from build123d import *

# Parameters (mm, degrees)
F0_W        = 127
F0_H        = 622.3
F1_DEPTH    = 19.05
F3_DEPTH    = 622.301
F5_D        = 12.7
F6_W        = 28.575
F6_H        = 28.575
F7_DEPTH    = 38.101
F8_C1_SIZE2 = 12.7
F8_C1_SIZE  = 3.175
F8_C2_SIZE2 = 3.175
F8_C2_SIZE  = 12.7


# Not quite as in the source:
# - a length typed as a fraction of an inch, garbled in the dataset ("3 / 203.2 mm" for 3/8 in), is restored
# - a pattern or mirror of a feature is missing from the dataset's text; its kind, count and spacing are read off the source's solid


with BuildPart() as f1:
    # F0 (on Front) → F1 (new body, symmetric)
    with BuildSketch(Plane.XZ):
        Rectangle(F0_W, F0_H)
    extrude(amount=F1_DEPTH, both=True)

    # F2 (on face) → F3 (cut, through all)
    with BuildSketch(Plane.XY.offset(311.15)):
        with BuildLine():
            ThreePointArc((-63.5, 2.159e-07), (-63.3181995898, 9.5319324627), (-62.773062814, 19.05))
            Line((-62.773062814, 19.05), (-63.5, 19.05))
            Line((-63.5, 19.05), (-63.5, 2.159e-07))
        make_face()
        with BuildLine():
            Line((-63.5, -19.05), (-62.773062814, -19.05))
            ThreePointArc((-62.773062814, -19.05), (-63.318199598, -9.531932247), (-63.5, 2.159e-07))
            Line((-63.5, 2.159e-07), (-63.5, -19.05))
        make_face()
    extrude(amount=-F3_DEPTH, mode=Mode.SUBTRACT)

    # F5 (through all)
    with Locations(Plane.XZ.offset(19.05)):
        with Locations((47.244, 177.8), (47.244, -215.9)):
            Hole(F5_D / 2)

    # F6 (on face) → F7 (cut, through all)
    with BuildSketch(Plane.XZ.offset(19.05)):
        with Locations((0.7239, 296.8625)):
            Rectangle(F6_W, F6_H)
    f7 = extrude(amount=-F7_DEPTH, mode=Mode.SUBTRACT)

    # F7_copies: F7 across plane
    add(f7.mirror(Plane(origin=(0, 0, 0), x_dir=(-1, 0, 0), z_dir=(0, 0, -1))), mode=Mode.SUBTRACT)

    # F8: chamfer of 12.7 x 3.175 on 2 edges, made by hand

    # F8_c1
    f8_c1_edges = [f1.edges().sort_by_distance(p)[0] for p in [
        (-63.5, 0, -311.15),
    ]]
    f8_c1_side = f1.faces().sort_by_distance((-63.4365, 0, -311.15))[0]
    chamfer(f8_c1_edges, length=F8_C1_SIZE, length2=F8_C1_SIZE2, reference=f8_c1_side)

    # F8_c2
    f8_c2_edges = [f1.edges().sort_by_distance(p)[0] for p in [
        (-63.5, 0, 311.15),
    ]]
    f8_c2_side = f1.faces().sort_by_distance((-63.5, 0, 311.0865))[0]
    chamfer(f8_c2_edges, length=F8_C2_SIZE, length2=F8_C2_SIZE2, reference=f8_c2_side)


solid = f1.part
Could you check a few things on this model? Use its own coordinates, in mm. A direction names the side the tool comes from. Give positions to 0.01 mm unless a question says otherwise; leave off trailing zeros. Write each loop counter-clockwise with the first axis right and the second up, starting at its lowest first coordinate (ties: lowest second). Pieces come first, ordered by that corner, then holes. Notation, with made-up numbers: (68.25, -20) -> (116.25, -20) arc R29 cw to (116.25, 16) -> close; hole circle Ø8 at (19.5, -11). An arc over 180 degrees is marked (long way). Write each question's results on one line, items separated by ' | '. Start each with the question number.
Q1. Suppose I cut it at C-C, the plane y = -9. State how many separate pieces and enclosed holes the cut face has, and give its area (3 significant figures).
Q2. I need wall thicknesses on probe 1 along X at (y, z) = (3, -215); probe 2 along Z at (x, y) = (-3, 7) (3 decimals); probe 3 along X at (y, z) = (7.5, 147.5). Which ranges of each line are inside material? Lowest first, please.
Q3. I'm going to push flat-ended pins straight in: pin 1 Ø8.5 at (x, y) = (3.5, 7) entering from -Z (3 decimals); pin 2 Ø8 at (x, y) = (-8, -10.5) entering from +Z (3 decimals). Where does each tip first touch, or does it pass through?
Q4. We'd pull the mould along X, two halves only. Please class faces 4 (the face through (1, 0, 282.575)), 5 (the face through (63.5, 0, -4)), 6 (the face through (-1, 19.05, 4)): +X half, -X half, draft (parallel to the pull), parting line (faces both ways), or undercut.
Q5. Suppose I cut it at A-A, the plane z = 177.8. List the corners of the cut face in (x, y) for me, and give its area (3 significant figures).
Q6. Suppose I cut it at B-B, the plane x = -0.5. List the corners of the cut face in (y, z) for me (3 decimals), and give its area (3 significant figures).
Q7. Which directions (+Z, -Z, +X, -X, +Y, -Y) give clear straight access to the entire face, cutting with the end or side of a thin tool? Please do faces 1 (the face through (15.011, 0, -297)), 2 (the face through (48.62, 0.27, -222.1)), 3 (the face through (-13.564, 0, 297)).
Outcome:
1) separate pieces: 1 | enclosed holes: 2 | area: 77,000 mm2
2) probe 1: -63.48 to 40.96, 53.53 to 63.5 | probe 2: -282.575 to 282.575 | probe 3: -63.39 to 63.5
3) pin 1: z = -282.575 | pin 2: z = 282.575
4) face 4: undercut | face 5: +X half | face 6: draft
5) outline: (-62.77, -19.05) -> (40.89, -19.05) -> (40.89, 19.05) -> (-62.77, 19.05) arc R249.97 ccw to start; (53.59, -19.05) -> (63.5, -19.05) -> (63.5, 19.05) -> (53.59, 19.05) -> close | area: 4,350 mm2
6) outline: (-19.05, -282.575) -> (19.05, -282.575) -> (19.05, 282.575) -> (-19.05, 282.575) -> close | area: 21,500 mm2
7) face 1: -Z, +Y, -Y | face 2: +Y, -Y | face 3: +Z, +Y, -Y
